Here's how the part is built. I have some questions about the finished solid (model axes, mm). A direction names the side the tool comes from. Round coordinates to 2 decimals unless told otherwise and drop trailing zeros. Write each loop counter-clockwise with the first axis right and the second up, starting at its lowest first coordinate (ties: lowest second). Pieces come first, ordered by that corner, then holes. Notation, with made-up numbers: M 40,-8 L 66,-8 A23 ccw 66,23 Z; hole C 61,11 d9. An arc over 180 degrees is marked long. Use one line per item in the form item = value. Start each with the question number.
Q1. I'm going to push flat-ended pins straight in: pin 1 Ø12 at (x, z) = (-14.5, 2) entering from +Y; pin 2 Ø2.5 at (y, z) = (3.5, -0.5) entering from -X; pin 3 Ø3 at (y, z) = (9.5, -0.5) entering from -X; pin 4 Ø3 at (x, y) = (9, 10) entering from -Z. Where does each tip first touch, or does it pass through?
Q2. I want a section at C-C on z = 11. List the corners of the cut face in (x, y) for me.
Q3. I want a section at B-B on x = 0. List the corners of the cut face in (y, z) for me.
Q4. For faces 1 (the face through (-10, 2.375, 0)), 2 (the face through (0.645, 10.486, 2.603)), 3 (the face through (16.726, 0, 0)), which set-ups out of +Z, -Z, +X, -X, +Y, -Y let a thin tool reach every point of the face, with its end or its side?
Q5. I want a section at D-D on x = 15. List the corners of the cut face in (y, z) for me.
Q6. I need wall thicknesses on line 1 along X through (y, z) = (5.5, 8.75); line 2 along Y through (x, z) = (0, -10.8); line 3 along Y through (x, z) = (0, 7.25). Which ranges of each line are inside material? Lowest first, please. Write a range as from..to.
Q7. I want a section at A-A on z = 8.25. List the corners of the cut face in (x, y) for me, and give its area (3 significant figures).
Q8. We'd pull the mould along X, two halves only. Please class faces 4 (the face through (19.05, 0, 0)), 5 (the face through (-16.726, 0, 0)), 6 (the face through (0, -2.375, 0)): +X half, -X half, draft (parallel to the pull), parting line (faces both ways), or undercut.
```python
from build123d import *

# Parameters (mm, degrees)
SKETCH1_R                      = 2.5527
BOSS_EXTRUDE1_DEPTH            = 12.7
FILLET1_R                      = 0.381
F_1_2_0_5_DIAMETER_HOLE2_D     = 9.906
F_1_2_0_5_DIAMETER_HOLE2_DEPTH = 19.05
F_1_2_0_5_DIAMETER_HOLE2_TIP   = 5.697774721
CHAMFER2_SIZE                  = 0.889
CUT_EXTRUDE1_DEPTH             = 9.906


with BuildPart() as part:
    # Sketch1 → Boss-Extrude1 (new, symmetric)
    with BuildSketch(Plane.XY):
        with BuildLine():
            Line((-19.05, -2.3749), (19.05, -2.3749))
            Line((19.05, -2.3749), (19.05, 2.3749))
            Line((19.05, 2.3749), (7.9248, 2.3749))
            Line((7.9248, 2.3749), (7.9248, 5.5753))
            ThreePointArc((7.9248, 5.5753), (0, 13.5001), (-7.9248, 5.5753))
            Line((-7.9248, 5.5753), (-7.9248, 2.3749))
            Line((-7.9248, 2.3749), (-19.05, 2.3749))
            Line((-19.05, 2.3749), (-19.05, -2.3749))
        make_face()
        with Locations((0, 5.5753)):
            Circle(SKETCH1_R, mode=Mode.SUBTRACT)
    extrude(amount=BOSS_EXTRUDE1_DEPTH, both=True)

    # Fillet1
    fillet1_edges = [part.edges().sort_by_distance(p)[0] for p in [
        (19.05, 2.3749, 0),
        (19.05, -2.3749, 0),
        (-19.05, -2.3749, 0),
        (-19.05, 2.3749, 0),
    ]]
    fillet(fillet1_edges, radius=FILLET1_R)

    # 1/2 (0.5) Diameter Hole2
    with Locations(Plane.XY.offset(12.7)):
        with Locations((0, 5.5753)):
            Hole(F_1_2_0_5_DIAMETER_HOLE2_D / 2, depth=F_1_2_0_5_DIAMETER_HOLE2_DEPTH)
            with Locations((0, 0, -(F_1_2_0_5_DIAMETER_HOLE2_DEPTH + F_1_2_0_5_DIAMETER_HOLE2_TIP / 2))):  # 82° drill point
                Cone(0, F_1_2_0_5_DIAMETER_HOLE2_D / 2, F_1_2_0_5_DIAMETER_HOLE2_TIP, mode=Mode.SUBTRACT)

    # Chamfer2
    chamfer2_edges = [part.edges().sort_by_distance(p)[0] for p in [
        (4.953, 5.5753, 12.7),
    ]]
    chamfer(chamfer2_edges, length=CHAMFER2_SIZE)

    # Sketch9 → Cut-Extrude1 (cut)
    with BuildSketch(Plane(origin=(0, 2.3749, 0), x_dir=(1, 0, 0), z_dir=(0, 1, 0))):
        with BuildLine():
            Line((16.7259, 6.35), (16.7259, -6.35))
            ThreePointArc((16.7259, -6.35), (13.4874, -9.5885), (10.2489, -6.35))
            Line((10.2489, -6.35), (10.2489, 6.35))
            ThreePointArc((10.2489, 6.35), (13.4874, 9.5885), (16.7259, 6.35))
        make_face()
        with BuildLine():
            Line((-16.7259, 6.35), (-16.7259, -6.35))
            ThreePointArc((-16.7259, -6.35), (-13.4874, -9.5885), (-10.2489, -6.35))
            Line((-10.2489, -6.35), (-10.2489, 6.35))
            ThreePointArc((-10.2489, 6.35), (-13.4874, 9.5885), (-16.7259, 6.35))
        make_face()
    extrude(amount=-CUT_EXTRUDE1_DEPTH, mode=Mode.SUBTRACT)


solid = part.part
```
Reported:
q1.pin_1 = 2.37
q1.pin_2 = -18.95
q1.pin_3 = -7.54
q1.pin_4 = through
q2.outline = M -19.05,-1.99 A0.38 ccw -18.67,-2.37 L 18.67,-2.37 A0.38 ccw 19.05,-1.99 L 19.05,1.99 A0.38 ccw 18.67,2.37 L 7.92,2.37 L 7.92,5.58 A7.92 ccw -7.92,5.58 L -7.92,2.37 L -18.67,2.37 A0.38 ccw -19.05,1.99 Z; hole C 0,5.58 d9.91
q3.outline = M -2.37,-12.7 L 3.02,-12.7 L 3.02,-9.11 L 0.62,-6.35 L 0.62,11.81 L -0.27,12.7 L -2.37,12.7 Z; M 8.13,-12.7 L 13.5,-12.7 L 13.5,12.7 L 11.42,12.7 L 10.53,11.81 L 10.53,-6.35 L 8.13,-9.11 Z
q4.face_1 = +Z, -Z, -X, +Y
q4.face_2 = +Z
q4.face_3 = +Y, -Y
q5.outline = M -2.37,-12.7 L 2.37,-12.7 L 2.37,-9.21 L -2.37,-9.21 Z; M -2.37,9.21 L 2.37,9.21 L 2.37,12.7 L -2.37,12.7 Z
q6.line_1 = -7.92..-4.95, 4.95..7.92
q6.line_2 = -2.37..3.02, 8.13..13.5
q6.line_3 = -2.37..0.62, 10.53..13.5
q7.outline = M -19.05,-1.99 A0.38 ccw -18.67,-2.37 L -16.11,-2.37 L -16.11,2.37 L -18.67,2.37 A0.38 ccw -19.05,1.99 Z; M -10.86,-2.37 L 10.86,-2.37 L 10.86,2.37 L 7.92,2.37 L 7.92,5.58 A7.92 ccw -7.92,5.58 L -7.92,2.37 L -10.86,2.37 Z; M 16.11,-2.37 L 18.67,-2.37 A0.38 ccw 19.05,-1.99 L 19.05,1.99 A0.38 ccw 18.67,2.37 L 16.11,2.37 Z; hole C 0,5.58 d9.91
q7.area = 203 mm^2
q8.face_4 = +X half
q8.face_5 = undercut
q8.face_6 = draft
